CAD build for the part. Positions are in the model's coordinates, mm. Face numbers are marked on the shaded views. Coordinates: 2 decimals unless noted, no trailing zeros. Loops run counter-clockwise (first coordinate to the right, second up) from the corner with the lowest first, then second, coordinate; pieces in that order, holes last. Notation, with made-up numbers: (83, 75.25) -> (122, 75.25) arc R24 ccw to (122, 89.25) -> close; hole circle Ø2 at (-15, 14.5). An arc over 180 degrees is marked (long way). Write item = value, one per line. Start each with the question number.
(1) Band-saw the part on A-A (x = 0). Write the cut outline in (y, z), and give its area (3 significant figures).
(2) Band-saw the part on D-D (x = -4.5). Write the cut outline in (y, z), and give its area (3 significant figures).
(3) Band-saw the part on B-B (z = -1). Write the cut outline in (x, y), and give its area (3 significant figures).
(4) Band-saw the part on C-C (x = 11.75). Write the cut outline in (y, z), and give its area (3 significant figures).
(5) Pull direction X, two halves, no side cores. Call the marked faces 1, 2 and 3: +X half, -X half, draft (parallel to the pull), parting line (faces both ways), or undercut.
(6) Flat gauge pins, fed straight in: P1, Ø1.5, axis at y = -6, z = 27, coming from the +X side; P2, Ø3, axis at y = -3.5, z = 24, coming from the -X side; P3, Ø8, axis at x = -0.5, z = -17.5, coming from the -Y side. Where does each tip first touch, or does it go through?
(7) Drill centre lines: line 1 (Z direction, x = 0, y = -4); line 2 (Z direction, x = 4, y = -3.5); line 3 (X direction, y = -3.75, z = 18). Where is each one in solid material? Low to high. Write a range as from..to.
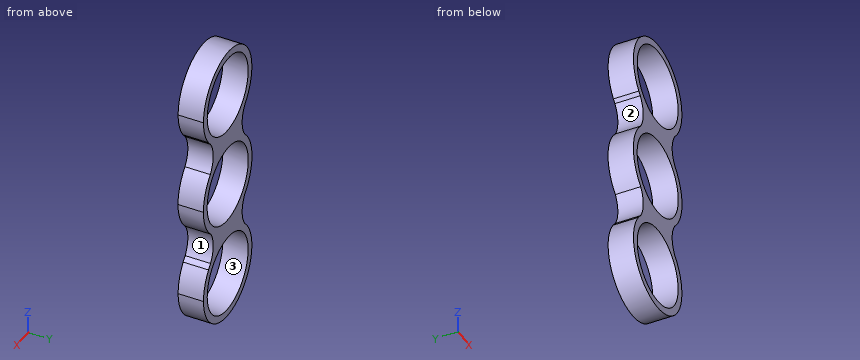
```python
from build123d import *

# Parameters (mm, degrees)
F0_R     = 11
F0_R_2   = 10.95
F1_DEPTH = 7


with BuildPart() as f1:
    # F0 (on Front) → F1 (new body)
    with BuildSketch(Plane.XZ):
        with BuildLine():
            ThreePointArc((9.079472, -9.303934), (11.97984, -5.048112), (13, 0))
            ThreePointArc((13, 0), (12.033855, 4.917961), (9.279025, 9.104927))
            ThreePointArc((9.279025, 9.104927), (0.140912, 12.999236), (-9.079472, 9.303934))
            ThreePointArc((-9.079472, 9.303934), (-13, 0), (-9.079472, -9.303934))
            ThreePointArc((-9.079472, -9.303934), (0, -13), (9.079472, -9.303934))
        make_face()
        Circle(F0_R, mode=Mode.SUBTRACT)
        with BuildLine():
            ThreePointArc((-9.079472, 9.303934), (0.140912, 12.999236), (9.279025, 9.104927))
            ThreePointArc((9.279025, 9.104927), (7.748031, 13.701905), (9.191158, 18.32722))
            ThreePointArc((9.191158, 18.32722), (-0.088011, 14.500299), (-9.314307, 18.45299))
            ThreePointArc((-9.314307, 18.45299), (-7.735521, 13.915972), (-9.079472, 9.303934))
        make_face()
        with BuildLine():
            ThreePointArc((9.173578, -18.259543), (7.733358, -13.796378), (9.079472, -9.303934))
            ThreePointArc((9.079472, -9.303934), (0, -13), (-9.079472, -9.303934))
            ThreePointArc((-9.079472, -9.303934), (-7.733358, -13.796378), (-9.173578, -18.259543))
            ThreePointArc((-9.173578, -18.259543), (0, -14.45), (9.173578, -18.259543))
        make_face()
        with BuildLine():
            ThreePointArc((10.26943, 19.560684), (9.698205, 18.972004), (9.191158, 18.32722))
            ThreePointArc((9.191158, 18.32722), (9.74982, 18.926883), (10.26943, 19.560684))
        make_face()
        with BuildLine():
            ThreePointArc((-9.314307, 18.45299), (-0.088011, 14.500299), (9.191158, 18.32722))
            ThreePointArc((9.191158, 18.32722), (9.698205, 18.972004), (10.26943, 19.560684))
            ThreePointArc((10.26943, 19.560684), (12.261558, 23.283864), (12.95, 27.45))
            ThreePointArc((12.95, 27.45), (-4.283246, 39.671142), (-10.116611, 19.365652))
            ThreePointArc((-10.116611, 19.365652), (-9.697869, 18.924783), (-9.314307, 18.45299))
        make_face()
        with Locations((0, 27.45)):
            Circle(F0_R_2, mode=Mode.SUBTRACT)
        with BuildLine():
            ThreePointArc((10.26943, -19.510684), (9.688458, -18.914058), (9.173578, -18.259543))
            ThreePointArc((9.173578, -18.259543), (0, -14.45), (-9.173578, -18.259543))
            ThreePointArc((-9.173578, -18.259543), (-9.688458, -18.914058), (-10.26943, -19.510684))
            ThreePointArc((-10.26943, -19.510684), (-4.166136, -39.661558), (12.95, -27.4))
            ThreePointArc((12.95, -27.4), (12.261558, -23.233864), (10.26943, -19.510684))
        make_face()
        with Locations((0, -27.4)):
            Circle(F0_R_2, mode=Mode.SUBTRACT)
        with BuildLine():
            ThreePointArc((10.26943, -19.510684), (9.741611, -18.867502), (9.173578, -18.259543))
            ThreePointArc((9.173578, -18.259543), (9.688458, -18.914058), (10.26943, -19.510684))
        make_face()
        with BuildLine():
            ThreePointArc((-10.116611, 19.365652), (-9.72617, 18.899905), (-9.314307, 18.45299))
            ThreePointArc((-9.314307, 18.45299), (-9.697869, 18.924783), (-10.116611, 19.365652))
        make_face()
        with BuildLine():
            ThreePointArc((-10.26943, -19.510684), (-9.688458, -18.914058), (-9.173578, -18.259543))
            ThreePointArc((-9.173578, -18.259543), (-9.741611, -18.867502), (-10.26943, -19.510684))
        make_face()
    extrude(amount=F1_DEPTH)


solid = f1.part
```
Findings below:
q1.outline = (-7, -40.35) -> (0, -40.35) -> (0, -38.35) -> (-7, -38.35) -> close; (-7, -16.45) -> (0, -16.45) -> (0, -11) -> (-7, -11) -> close; (-7, 11) -> (0, 11) -> (0, 16.5) -> (-7, 16.5) -> close; (-7, 38.4) -> (0, 38.4) -> (0, 40.4) -> (-7, 40.4) -> close
q1.area = 105 mm²
q2.outline = (-7, -39.54) -> (0, -39.54) -> (0, -37.38) -> (-7, -37.38) -> close; (-7, -17.42) -> (0, -17.42) -> (0, -10.04) -> (-7, -10.04) -> close; (-7, 10.04) -> (0, 10.04) -> (0, 17.47) -> (-7, 17.47) -> close; (-7, 37.43) -> (0, 37.43) -> (0, 39.59) -> (-7, 39.59) -> close
q2.area = 134 mm²
q3.outline = (-12.96, -7) -> (-10.95, -7) -> (-10.95, 0) -> (-12.96, 0) -> close; (10.95, -7) -> (12.96, -7) -> (12.96, 0) -> (10.95, 0) -> close
q3.area = 28.1 mm²
q4.outline = (-7, -32.84) -> (0, -32.84) -> (0, -21.96) -> (-7, -21.96) -> close; (-7, -5.56) -> (0, -5.56) -> (0, 5.56) -> (-7, 5.56) -> close; (-7, 22.01) -> (0, 22.01) -> (0, 32.89) -> (-7, 32.89) -> close
q4.area = 230 mm²
q5.face_1 = +X half
q5.face_2 = -X half
q5.face_3 = undercut
q6.P1 = 12.95
q6.P2 = -12.8
q6.P3 = -7
q7.line_1 = -40.35..-38.35, -16.45..-11, 11..16.5, 38.4..40.4
q7.line_2 = -39.72..-37.59, -17.21..-10.25, 10.25..17.26, 37.64..39.77
q7.line_3 = -9..-5.53, 5.53..8.97
